from build123d import *

# Parameters (mm, degrees)
PAD067_DEPTH    = 14.85
SKETCH113_W     = 92.842344
SKETCH113_H     = 21.437685
SKETCH113_W_2   = 28.846216
SKETCH113_H_2   = 21.567847
POCKET027_DEPTH = 22.351
SKETCH114_R     = 3
PAD068_DEPTH    = 9.85


with BuildPart() as part:
    # Sketch112 (on DatumPlane) → Pad067 (new body)
    with BuildSketch(Plane.XY.offset(1.6)):
        Polygon((47, 111), (153.5, 111), (171.2268158449, 89.65), (171.2268158449, 88.65), (52.4768158449, 88.65), (47, 90.5590542687), align=None)
    extrude(amount=PAD067_DEPTH)

    # Sketch113 (on Face4 of Pad067) → Pocket027 (cut, through all)
    with BuildSketch(Plane(origin=(0, 88.65, 1.6), x_dir=(1, 0, 0), z_dir=(0, -1, 0))):
        with Locations((88.078828, -0.8688425)):
            Rectangle(SKETCH113_W, SKETCH113_H)
        with Locations((158.923108, 2.4660765)):
            Rectangle(SKETCH113_W_2, SKETCH113_H_2)
    extrude(amount=-POCKET027_DEPTH, mode=Mode.SUBTRACT)

    # Sketch114 (on Face2 of Pocket027) → Pad068 (join)
    with BuildSketch(Plane(origin=(0, 0, 11.45), x_dir=(1, 0, 0), z_dir=(0, 0, -1))):
        with Locations((61, -100)):
            Circle(SKETCH114_R)
    extrude(amount=PAD068_DEPTH)


solid = part.part
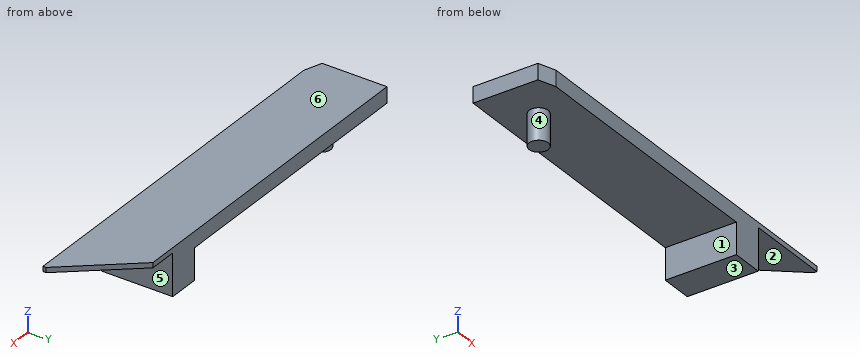
Read the model definition and answer for the solid it produces. Units are mm, in the model's axes. Face numbers are marked on the shaded views. A direction names the side the tool comes from. Coordinates: 2 decimals unless noted, no trailing zeros. Order: outer loops, then holes, each group sorted by start corner. A loop starts at its lowest first (then second) coordinate and runs counter-clockwise, first axis right, second up. Notation, with made-up numbers: (49, -16.5) - (56, -16.5) arc R18 ccw to (56, -0.5) - close; hole circle Ø4 at (59.25, 73). An arc over 180 degrees is marked (long way). Use one line per item in the form item = value.
(1) Section B-B, the plane z = 5.5 is taken. Give the vertices of the cut face in (x, y).
Computed values:
outline = circle Ø6 at (61, 100); (134.5, 88.65) - (144.5, 88.65) - (144.5, 111) - (134.5, 111) - close
(2) Straight lines are drawn through the part: L1, parallel to X at y = 104.5, z = 13.5; L2, parallel to Z at x = 97, y = 106; L3, parallel to X at y = 100.25, z = 3. For each, find the intervals that lie inside material, in ascending order.
Computed values:
L1 = 47 to 144.5
L2 = 11.45 to 16.45
L3 = 58.01 to 63.99, 134.5 to 144.5
(3) Which of the six approach directions +Z, -Z, +X, -X, +Y, -Y give full straight-line access (tool end or side, diameter ignored) to the marked faces 1, 2 and 3?
Computed values:
face_1 = -Z, +Y, -Y
face_2 = -Z, +X, +Y, -Y
face_3 = -Z, +X, -X, +Y, -Y
(4) Section D-D, the plane z = 13.5 is taken. Give the vertices of the cut face in (x, y), then the cut area to 3 significant figures.
Computed values:
outline = (47, 90.56) - (52.48, 88.65) - (144.5, 88.65) - (144.5, 111) - (47, 111) - close
area = 2,170 mm²
(5) Section C-C, the plane y = 93.5 is taken. Give the vertices of the cut face in (x, z), then the cut area to 3 significant figures.
Computed values:
outline = (47, 11.45) - (134.5, 11.45) - (134.5, 1.6) - (144.5, 1.6) - (144.5, 14.85) - (168.03, 14.85) - (168.03, 16.45) - (47, 16.45) - close
area = 624 mm²
(6) For a pull along X with two mould halves and no side action, classify the marked faces 4, 5 and 6 as pulls with the +X half, pulls with the -X half, needs draft (parallel to the pull), parting line crosses it, or undercut.
Computed values:
face_4 = undercut
face_5 = pulls with the +X half
face_6 = needs draft
(7) Given pin 1 Ø6 at (x, y) = (73.5, 94.5) entering from -Z; pin 2 Ø3 at (x, y) = (158, 106) entering from -Z, each flat-ended and moving along its own axis, determine where each tip first touches the part or whether it passes through.
Computed values:
pin_1 = 11.45
pin_2 = 14.85
(8) Section A-A, the plane x = 61 is taken. Give the vertices of the cut face in (y, z).
Computed values:
outline = (88.65, 11.45) - (97, 11.45) - (97, 1.6) - (103, 1.6) - (103, 11.45) - (111, 11.45) - (111, 16.45) - (88.65, 16.45) - close
